```python
from build123d import *

# Parameters (mm, degrees)
SKETCH_1_R      = 1.25
SKETCH_1_R_2    = 1
EXTRUDE_3_DEPTH = 2


with BuildPart() as part:
    # 草圖1 → 填料-伸長3 (new body)
    with BuildSketch(Plane.XY):
        with BuildLine():
            Line((-53.694067148, 36.989902751), (-54.694067148, 36.989902751))
            Line((-54.694067148, 36.989902751), (-54.694067148, 35.989902751))
            Line((-54.694067148, 35.989902751), (-54.694067148, -10.010097249))
            Line((-54.694067148, -10.010097249), (-54.694067148, -11.010097249))
            Line((-54.694067148, -11.010097249), (-53.694067148, -11.010097249))
            Line((-53.694067148, -11.010097249), (-46.694067148, -11.010097249))
            Line((-46.694067148, -11.010097249), (-46.694067148, -9.010097249))
            ThreePointArc((-46.694067148, -9.010097249), (-46.401173929, -8.302990468), (-45.694067148, -8.010097249))
            Line((-45.694067148, -8.010097249), (-43.694067148, -8.010097249))
            ThreePointArc((-43.694067148, -8.010097249), (-42.986960367, -8.302990468), (-42.694067148, -9.010097249))
            Line((-42.694067148, -9.010097249), (-42.694067148, -11.010097249))
            Line((-42.694067148, -11.010097249), (-34.694067148, -11.010097249))
            Line((-34.694067148, -11.010097249), (-34.694067148, -9.010097249))
            ThreePointArc((-34.694067148, -9.010097249), (-34.401173929, -8.302990468), (-33.694067148, -8.010097249))
            Line((-33.694067148, -8.010097249), (-31.694067148, -8.010097249))
            ThreePointArc((-31.694067148, -8.010097249), (-30.986960367, -8.302990468), (-30.694067148, -9.010097249))
            Line((-30.694067148, -9.010097249), (-30.694067148, -11.010097249))
            Line((-30.694067148, -11.010097249), (17.305932852, -11.010097249))
            Line((17.305932852, -11.010097249), (17.305932852, -9.010097249))
            ThreePointArc((17.305932852, -9.010097249), (17.598826071, -8.302990468), (18.305932852, -8.010097249))
            Line((18.305932852, -8.010097249), (20.305932852, -8.010097249))
            ThreePointArc((20.305932852, -8.010097249), (21.013039633, -8.302990468), (21.305932852, -9.010097249))
            Line((21.305932852, -9.010097249), (21.305932852, -11.010097249))
            Line((21.305932852, -11.010097249), (29.305932852, -11.010097249))
            Line((29.305932852, -11.010097249), (29.305932852, -9.010097249))
            ThreePointArc((29.305932852, -9.010097249), (29.598826071, -8.302990468), (30.305932852, -8.010097249))
            Line((30.305932852, -8.010097249), (32.305932852, -8.010097249))
            ThreePointArc((32.305932852, -8.010097249), (33.013039633, -8.302990468), (33.305932852, -9.010097249))
            Line((33.305932852, -9.010097249), (33.305932852, -11.010097249))
            Line((33.305932852, -11.010097249), (40.305932852, -11.010097249))
            Line((40.305932852, -11.010097249), (41.305932852, -11.010097249))
            Line((41.305932852, -11.010097249), (41.305932852, -10.010097249))
            Line((41.305932852, -10.010097249), (41.305932852, 35.989902751))
            Line((41.305932852, 35.989902751), (41.305932852, 36.989902751))
            Line((41.305932852, 36.989902751), (40.305932852, 36.989902751))
            Line((40.305932852, 36.989902751), (-53.694067148, 36.989902751))
        make_face()
        with Locations((-20.194067148, 23.489902751)):
            Circle(SKETCH_1_R, mode=Mode.SUBTRACT)
        with Locations((6.805932852, 23.489902751)):
            Circle(SKETCH_1_R, mode=Mode.SUBTRACT)
        with Locations((6.805932852, -6.510097249)):
            Circle(SKETCH_1_R, mode=Mode.SUBTRACT)
        with Locations((-20.194067148, -6.510097249)):
            Circle(SKETCH_1_R, mode=Mode.SUBTRACT)
        with Locations((27.305932852, 28.989902751)):
            Circle(SKETCH_1_R_2, mode=Mode.SUBTRACT)
        with Locations((-48.694067148, 28.989902751)):
            Circle(SKETCH_1_R_2, mode=Mode.SUBTRACT)
        with Locations((-28.694067148, 34.989902751)):
            Circle(SKETCH_1_R_2, mode=Mode.SUBTRACT)
        with Locations((-36.694067148, 28.989902751)):
            Circle(SKETCH_1_R_2, mode=Mode.SUBTRACT)
        with Locations((-28.694067148, -7.010097249)):
            Circle(SKETCH_1_R_2, mode=Mode.SUBTRACT)
        with Locations((15.305932852, 34.989902751)):
            Circle(SKETCH_1_R_2, mode=Mode.SUBTRACT)
        with Locations((-28.694067148, 28.989902751)):
            Circle(SKETCH_1_R_2, mode=Mode.SUBTRACT)
        with Locations((-36.694067148, -7.010097249)):
            Circle(SKETCH_1_R_2, mode=Mode.SUBTRACT)
        with Locations((-40.694067148, -7.010097249)):
            Circle(SKETCH_1_R_2, mode=Mode.SUBTRACT)
        with Locations((-48.694067148, -7.010097249)):
            Circle(SKETCH_1_R_2, mode=Mode.SUBTRACT)
        with Locations((35.305932852, -7.010097249)):
            Circle(SKETCH_1_R_2, mode=Mode.SUBTRACT)
        with Locations((-40.694067148, 28.989902751)):
            Circle(SKETCH_1_R_2, mode=Mode.SUBTRACT)
        with Locations((27.305932852, -7.010097249)):
            Circle(SKETCH_1_R_2, mode=Mode.SUBTRACT)
        with Locations((23.305932852, -7.010097249)):
            Circle(SKETCH_1_R_2, mode=Mode.SUBTRACT)
        with Locations((15.305932852, 28.989902751)):
            Circle(SKETCH_1_R_2, mode=Mode.SUBTRACT)
        with Locations((15.305932852, -7.010097249)):
            Circle(SKETCH_1_R_2, mode=Mode.SUBTRACT)
        with Locations((23.305932852, 28.989902751)):
            Circle(SKETCH_1_R_2, mode=Mode.SUBTRACT)
        with Locations((35.305932852, 28.989902751)):
            Circle(SKETCH_1_R_2, mode=Mode.SUBTRACT)
        with BuildLine():
            Line((-14.194067148, 31.989902751), (0.805932852, 31.989902751))
            ThreePointArc((0.805932852, 31.989902751), (1.513039633, 31.697009532), (1.805932852, 30.989902751))
            Line((1.805932852, 30.989902751), (1.805932852, 17.989902751))
            ThreePointArc((1.805932852, 17.989902751), (1.513039633, 17.28279597), (0.805932852, 16.989902751))
            Line((0.805932852, 16.989902751), (-14.194067148, 16.989902751))
            ThreePointArc((-14.194067148, 16.989902751), (-14.901173929, 17.28279597), (-15.194067148, 17.989902751))
            Line((-15.194067148, 17.989902751), (-15.194067148, 30.989902751))
            ThreePointArc((-15.194067148, 30.989902751), (-14.901173929, 31.697009532), (-14.194067148, 31.989902751))
        make_face(mode=Mode.SUBTRACT)
        with BuildLine():
            Line((-46.694067148, 30.989902751), (-46.694067148, 32.989902751))
            ThreePointArc((-46.694067148, 32.989902751), (-46.401173929, 33.697009532), (-45.694067148, 33.989902751))
            Line((-45.694067148, 33.989902751), (-43.694067148, 33.989902751))
            ThreePointArc((-43.694067148, 33.989902751), (-42.986960367, 33.697009532), (-42.694067148, 32.989902751))
            Line((-42.694067148, 32.989902751), (-42.694067148, 30.989902751))
            ThreePointArc((-42.694067148, 30.989902751), (-42.986960367, 30.28279597), (-43.694067148, 29.989902751))
            Line((-43.694067148, 29.989902751), (-45.694067148, 29.989902751))
            ThreePointArc((-45.694067148, 29.989902751), (-46.401173929, 30.28279597), (-46.694067148, 30.989902751))
        make_face(mode=Mode.SUBTRACT)
        with BuildLine():
            Line((-30.694067148, 30.989902751), (-30.694067148, 32.989902751))
            ThreePointArc((-30.694067148, 32.989902751), (-30.986960367, 33.697009532), (-31.694067148, 33.989902751))
            Line((-31.694067148, 33.989902751), (-33.694067148, 33.989902751))
            ThreePointArc((-33.694067148, 33.989902751), (-34.401173929, 33.697009532), (-34.694067148, 32.989902751))
            Line((-34.694067148, 32.989902751), (-34.694067148, 30.989902751))
            ThreePointArc((-34.694067148, 30.989902751), (-34.401173929, 30.28279597), (-33.694067148, 29.989902751))
            Line((-33.694067148, 29.989902751), (-31.694067148, 29.989902751))
            ThreePointArc((-31.694067148, 29.989902751), (-30.986960367, 30.28279597), (-30.694067148, 30.989902751))
        make_face(mode=Mode.SUBTRACT)
        with BuildLine():
            Line((20.305932852, 33.989902751), (18.305932852, 33.989902751))
            ThreePointArc((18.305932852, 33.989902751), (17.598826071, 33.697009532), (17.305932852, 32.989902751))
            Line((17.305932852, 32.989902751), (17.305932852, 30.989902751))
            ThreePointArc((17.305932852, 30.989902751), (17.598826071, 30.28279597), (18.305932852, 29.989902751))
            Line((18.305932852, 29.989902751), (20.305932852, 29.989902751))
            ThreePointArc((20.305932852, 29.989902751), (21.013039633, 30.28279597), (21.305932852, 30.989902751))
            Line((21.305932852, 30.989902751), (21.305932852, 32.989902751))
            ThreePointArc((21.305932852, 32.989902751), (21.013039633, 33.697009532), (20.305932852, 33.989902751))
        make_face(mode=Mode.SUBTRACT)
        with BuildLine():
            Line((32.305932852, 29.989902751), (30.305932852, 29.989902751))
            ThreePointArc((30.305932852, 29.989902751), (29.598826071, 30.28279597), (29.305932852, 30.989902751))
            Line((29.305932852, 30.989902751), (29.305932852, 32.989902751))
            ThreePointArc((29.305932852, 32.989902751), (29.598826071, 33.697009532), (30.305932852, 33.989902751))
            Line((30.305932852, 33.989902751), (32.305932852, 33.989902751))
            ThreePointArc((32.305932852, 33.989902751), (33.013039633, 33.697009532), (33.305932852, 32.989902751))
            Line((33.305932852, 32.989902751), (33.305932852, 30.989902751))
            ThreePointArc((33.305932852, 30.989902751), (33.013039633, 30.28279597), (32.305932852, 29.989902751))
        make_face(mode=Mode.SUBTRACT)
    extrude(amount=EXTRUDE_3_DEPTH)


solid = part.part
```
The listing builds one solid part. Answer for the finished solid, in the listing's coordinates (mm). A direction names the side the tool comes from. Coordinates: 2 decimals unless noted, no trailing zeros. Loops run counter-clockwise (first coordinate to the right, second up) from the corner with the lowest first, then second, coordinate; pieces in that order, holes last. Notation, with made-up numbers: M -36.5,51 L 1.5,51 A25 cw 1.5,66 Z; hole C 12,52 d7. An arc over 180 degrees is marked long. Answer as CSV lines item,"result". Start each with the question number.
(1) Find the intervals of material crossed by L1, parallel to Y at x = 18.5, z = 1.7; L2, parallel to X at y = 25, z = 1.05; L3, parallel to Y at x = 6, z = 0.5, in increasing order. Write a range as [from, to].
(2) The mould has two halves that part along X. Classify faces 1 (the flat face through (25, -11.01, 1)), 2 (the cylindrical face through (14.5, -7.6, 1)), 3 (the cylindrical face through (-37.4, 29.7, 1)): pulls with the +X half, pulls with the -X half, needs draft (parallel to the pull), parting line crosses it, or undercut.
(3) The part is cut by section A-A (x = -3.5). Give the vertices of the cut face in (y, z), and give its area (3 significant figures).
(4) For faces 4 (the flat face through (-7, 13, 0)), 5 (the flat face through (-42.694, -10, 1)), 6 (the flat face through (-7, 16.99, 1)), determine the directions among +Z, -Z, +X, -X, +Y, -Y from which every point of the face is accessible in a straight line to the end or side of a thin tool.
(5) The part is cut by section B-B (z = 0.7). State how many separate pieces and enclosed holes the cut face has, and give its area (3 significant figures).
(6) Given pin 1 (1.6 mm diameter, centred on x = 15.31, y = 28.99, fed in from -Z); pin 2 (1 mm diameter, centred on x = -32.5, z = 1, fed in from -Y), each flat-ended and moving along its own axis, determine where each tip first touches the part or whether it passes through.
Determined:
1,L1,"[-8.01, 29.99], [33.99, 36.99]"
1,L2,"[-54.69, -15.19], [1.81, 41.31]"
1,L3,"[-11.01, -7.47], [-5.55, 22.53], [24.45, 36.99]"
2,face 1,"needs draft"
2,face 2,"undercut"
2,face 3,"undercut"
3,outline,"M -11.01,0 L 16.99,0 L 16.99,2 L -11.01,2 Z; M 31.99,0 L 36.99,0 L 36.99,2 L 31.99,2 Z"
3,area,"66.0 mm2"
4,face 4,"-Z, +X, -X, +Y, -Y"
4,face 5,"+Z, -Z, -Y"
4,face 6,"+Z, -Z"
5,separate pieces,"1"
5,enclosed holes,"27"
5,area,"4,170 mm2"
6,pin 1,"through"
6,pin 2,"y = -8.01"
